```python
from build123d import *

# Parameters (mm, degrees)
HEX_CUT_DEPTH = 3.175


with BuildPart() as part:
    # Sketch1 → Screw revolve (revolve)
    with BuildSketch(Plane.XY, mode=Mode.PRIVATE) as screw_revolve_sk:
        with BuildLine():
            Line((0, 0), (3.96875, 0))
            Line((3.96875, 0), (3.96875, 15.875))
            Line((3.96875, 15.875), (8.5725, 15.875))
            Line((8.5725, 15.875), (8.5725, 17.145))
            Line((8.5725, 17.145), (6.35, 17.145))
            ThreePointArc((6.35, 17.145), (4.822276438, 19.036685873), (2.756963005, 20.32))
            Line((2.756963005, 20.32), (0, 20.32))
            Line((0, 20.32), (0, 0))
        make_face()
    revolve(screw_revolve_sk.sketch.rotate(Axis((0, 0, 0), (0, 1, 0)), 90), axis=Axis((0, 0, 0), (0, 1, 0)))

    # Sketch2 → Hex Cut (cut)
    with BuildSketch(Plane(origin=(0, 20.32, 0), x_dir=(-1, 0, 0), z_dir=(0, 1, 0))):
        Polygon((-2.756963005, 0), (-1.378481503, -2.3876), (1.378481503, -2.3876), (2.756963005, 0), (1.378481503, 2.3876), (-1.378481503, 2.3876), align=None)
    extrude(amount=-HEX_CUT_DEPTH, mode=Mode.SUBTRACT)


solid = part.part
```
CAD build for the part. Positions are in the model's coordinates, mm. A direction names the side the tool comes from. Give positions to 0.01 mm unless a question says otherwise; leave off trailing zeros. Loops run counter-clockwise (first coordinate to the right, second up) from the corner with the lowest first, then second, coordinate; pieces in that order, holes last. Notation, with made-up numbers: M 49,38.5 L 103,38.5 A21 ccw 103,63.5 Z; hole C 2,35 d5. An arc over 180 degrees is marked long. Use one line per item in the form item = value.
Item 1: Flat gauge pins, fed straight in: pin 1 (2 mm diameter, centred on x = 0, y = 19, fed in from +Z); pin 2 (10 mm diameter, centred on x = -5.5, y = 6.5, fed in from -Z); pin 3 (8 mm diameter, centred on x = -1.5, y = 10.5, fed in from -Z). Where does each tip first touch, or does it go through?
Determined:
pin_1 = 5.79
pin_2 = -3.94
pin_3 = -3.97
Item 2: Which spindle directions (+Z, -Z, +X, -X, +Y, -Y) get a long thin tool onto all of the face, cutting with end or side? Do faces 1 (the face through (2, 15.875, 4)), 2 (the face through (3, 17.145, 6)), 3 (the face through (-2.57, 16.52, -8.18)). Say none if no direction does.
Determined:
face_1 = -Y
face_2 = +Y
face_3 = +Y, -Y
Item 3: Drill centre lines: probe 1 along Y at (x, z) = (-3, 8) (3 decimals); probe 2 along X at (y, z) = (18.5, 1); probe 3 along Y at (x, z) = (-0.25, 0) (3 decimals). Where is each one in solid material? Low to high. Write a range as from..to.
Determined:
probe_1 = 15.875..17.145
probe_2 = -5.27..-2.18, 2.18..5.27
probe_3 = 0..17.145
Item 4: Slice it at B-B (z = 3.25). List the corners of the cut face in (x, y) (3 decimals).
Determined:
outline = M -7.933,15.875 L -2.278,15.875 L -2.278,0 L 2.278,0 L 2.278,15.875 L 7.933,15.875 L 7.933,17.145 L 5.455,17.145 A6.517 ccw -5.455,17.145 L -7.933,17.145 Z
Item 5: Slice it at D-D (z = 1.5). List the corners of the cut face in (x, y) (3 decimals).
Determined:
outline = M -8.44,15.875 L -3.674,15.875 L -3.674,0 L 3.674,0 L 3.674,15.875 L 8.44,15.875 L 8.44,17.145 L 6.17,17.145 A7.126 ccw 2.313,20.32 L 1.891,20.32 L 1.891,17.145 L -1.891,17.145 L -1.891,20.32 L -2.313,20.32 A7.126 ccw -6.17,17.145 L -8.44,17.145 Z
Item 6: Slice it at C-C (y = 4.5). List the corners of the cut face in (x, z).
Determined:
outline = C 0,0 d7.94
Item 7: Two-plate mould, pull along Z, no slides. Class faces 4 (the face through (3.874, 8.049, 0.86)), 5 (the face through (0, 0, 0)), 6 (the face through (0, 19, 2.388)): pulls with the +Z half, pulls with the -Z half, needs draft (parallel to the pull), parting line crosses it, or undercut.
Determined:
face_4 = parting line crosses it
face_5 = needs draft
face_6 = undercut
